Design review of the part built by this model. Coordinates are the model's own, in mm. A direction names the side the tool comes from. Give positions to 0.01 mm unless a question says otherwise; leave off trailing zeros. Write each loop counter-clockwise with the first axis right and the second up, starting at its lowest first coordinate (ties: lowest second). Pieces come first, ordered by that corner, then holes. Notation, with made-up numbers: (88.5, -16) -> (99.5, -16) arc R18 ccw to (99.5, 2) -> close; hole circle Ø1 at (21.25, -24). An arc over 180 degrees is marked (long way). Answer as a JSON object with one key per item and string values.
Autodesk Inventor part; units mm, degrees
ref_plane "Arbeitsebene1" through (-21.4485, 99.4, 5.4) normal (-1, 0, 0) x (0, -0.6026, -0.798)
ref_plane "Arbeitsebene2" through (53.5515, 27.1, 8) normal (0, 0, -1) x (0, 1, 0)
ref_plane "YZ Plane" through (0, 0, 0) normal (1, 0, 0) x (0, 1, 0)
ref_plane "Arbeitsebene1" through (-21.4485, 99.4, 5.4) normal (-1, 0, 0) x (0, -0.6026, -0.798)
sketch "center1" plane through (-21.4485, 99.4, 5.4) normal (-1, 0, 0) x (0, -0.6026, -0.798)
  line L0 (125.8462, -4.4299) -> (-42.8597, 122.9603)
  line L1 (111.6965, 152.237) -> (-23.2865, -26.5243)
  point P0 (64.2081, 76.0713)
ref_plane "Arbeitsebene2" through (53.5515, 27.1, 8) normal (0, 0, -1) x (0, 1, 0)
sketch "center2" plane through (53.5515, 27.1, 8) normal (0, 0, -1) x (0, 1, 0)
  line L0 (0, 239.86) -> (0, -220.81)
  point P0 (-27.1, -53.5515)
sketch "Hallsensor" plane through (0, 0, 0) normal (0, 1, 0) x (-1, 0, 0)
  line L0 (21.4485, 13) -> (41.4485, 13) construction
  line L1 (41.4485, 13) -> (41.4485, 3) construction
  line L2 (41.4485, 3) -> (21.4485, 3) construction
  line L3 (21.4485, 3) -> (21.4485, 13) construction
  line L4 (21.4485, -97.7) -> (21.4485, 113.7) construction
  line L5 (-293.4115, 8) -> (167.2585, 8) construction
  line L6 (40.4485, 4) -> (42.4485, 4)
  line L7 (42.4485, 4) -> (42.4485, 2)
  line L8 (42.4485, 2) -> (40.4485, 2)
  line L9 (40.4485, 2) -> (40.4485, 4)
  line L10 (40.4485, 4) -> (42.4485, 2) construction
  line L11 (42.4485, 4) -> (40.4485, 2) construction
  line L12 (22.4485, 4) -> (20.4485, 4)
  line L13 (20.4485, 4) -> (20.4485, 2)
  line L14 (20.4485, 2) -> (22.4485, 2)
  line L15 (22.4485, 2) -> (22.4485, 4)
  line L16 (22.4485, 4) -> (20.4485, 2) construction
  line L17 (20.4485, 4) -> (22.4485, 2) construction
  line L18 (22.4485, 14) -> (20.4485, 14)
  line L19 (20.4485, 14) -> (20.4485, 12)
  line L20 (20.4485, 12) -> (22.4485, 12)
  line L21 (22.4485, 12) -> (22.4485, 14)
  line L22 (22.4485, 14) -> (20.4485, 12) construction
  line L23 (20.4485, 14) -> (22.4485, 12) construction
  line L24 (42.4485, 14) -> (40.4485, 14)
  line L25 (40.4485, 14) -> (40.4485, 12)
  line L26 (40.4485, 12) -> (42.4485, 12)
  line L27 (42.4485, 12) -> (42.4485, 14)
  line L28 (42.4485, 14) -> (40.4485, 12) construction
  line L29 (40.4485, 14) -> (42.4485, 12) construction
  line L30 (51.4485, -1) -> (1.4485, -1) construction
  line L31 (1.4485, -1) -> (1.4485, 17) construction
  line L32 (1.4485, 17) -> (51.4485, 17) construction
  line L33 (51.4485, 17) -> (51.4485, -1) construction
  circle A0 centre (51.4485, 8) radius 1.5
  circle A1 centre (1.4485, -1) radius 1.5
  circle A2 centre (1.4485, 17) radius 1.5
  point P0 (0, 0)
  point P1 (21.4485, 3)
  point P2 (21.4485, 3)
  dimension "d70" = 20
  dimension "d71" = 10
  dimension "d72" = 2
  dimension "d73" = 4
  dimension "d74" = 4
  dimension "d75" = 20
  dimension "d76" = 10
  dimension "d77" = 3
  dimension "d78" = 5
sketch "Groundplane" plane through (0, 0, 0) normal (0, 1, 0) x (-1, 0, 0)
  line L0 (-293.4115, 8) -> (167.2585, 8) construction
  line L1 (21.4485, -97.7) -> (21.4485, 113.7) construction
  arc A0 (22.4485, -32) -> (20.4485, -32) centre (21.4485, -32) ccw construction
  line L2 (22.4485, -32) -> (20.4485, -32) construction
  line L3 (20.4485, -32) -> (20.4485, -37) construction
  line L4 (20.4485, -37) -> (22.4485, -37) construction
  line L5 (22.4485, -37) -> (22.4485, -32) construction
  arc A1 (20.4485, 48) -> (22.4485, 48) centre (21.4485, 48) ccw construction
  line L6 (20.4485, 48) -> (22.4485, 48) construction
  line L7 (22.4485, 48) -> (22.4485, 53) construction
  line L8 (22.4485, 53) -> (20.4485, 53) construction
  line L9 (20.4485, 53) -> (20.4485, 48) construction
  line L10 (61.4485, -37) -> (-28.5515, -37) construction
  line L11 (-28.5515, -37) -> (-28.5515, 53) construction
  line L12 (-28.5515, 53) -> (61.4485, 53) construction
  line L13 (61.4485, 53) -> (61.4485, -37) construction
  dimension "d87" = 5
  dimension "d88" = 2
  dimension "d89" = 2
  dimension "d90" = 5
  dimension "d91" = 90
  dimension "d92" = 45
  dimension "d97" = 50
  dimension "d98" = 90
sketch "Montagepunkte" plane through (0, 0, 0) normal (0, 1, 0) x (-1, 0, 0)
  circle A0 centre (51.4485, 8) radius 1.5 construction
  circle A1 centre (1.4485, -1) radius 1.5 construction
  circle A2 centre (1.4485, 17) radius 1.5 construction
  line L0 (1.4485, -1) -> (-18.5515, -1) construction
  line L1 (-18.5515, -1) -> (-18.5515, 17) construction
  line L2 (-18.5515, 17) -> (1.4485, 17) construction
  line L3 (1.4485, 17) -> (1.4485, -1) construction
  line L4 (51.4485, 8) -> (31.4485, 8) construction
  circle A3 centre (31.4485, 8) radius 1.6
  circle A4 centre (51.4485, 8) radius 1.6
  circle A5 centre (1.4485, -1) radius 1.6
  circle A6 centre (1.4485, 17) radius 1.6
  circle A7 centre (-18.5515, 17) radius 1.6
  circle A8 centre (-18.5515, -1) radius 1.6
  arc A9 (22.4485, -32) -> (20.4485, -32) centre (21.4485, -32) ccw construction
  arc A10 (20.4485, 48) -> (22.4485, 48) centre (21.4485, 48) ccw construction
  circle A11 centre (21.4485, -32) radius 1
  circle A12 centre (21.4485, 48) radius 1
  dimension "d93" = 20
  dimension "d94" = 20
  dimension "d95" = 3.2
  dimension "d96" = 2
sketch "Skizze5" plane through (0, 0, 0) normal (0, 1, 0) x (-1, 0, 0)
  line L0 (-293.4115, 8) -> (167.2585, 8) construction
  circle A0 centre (21.4485, -32) radius 1
  circle A1 centre (21.4485, 48) radius 1
  line L1 (61.4485, -37) -> (-28.5515, -37)
  line L2 (61.4485, 53) -> (61.4485, -37)
  line L3 (-28.5515, -37) -> (-28.5515, 53)
  line L4 (-28.5515, 53) -> (61.4485, 53)
extrude "Extrusion2" add sketch "Skizze5" along normal blind 5
sketch "Skizze6" plane through (0, 5, 0) normal (0, 1, 0) x (1, 0, 0)
  line L0 (-56.4485, -3) -> (-26.4485, -3)
  line L1 (-26.4485, -3) -> (-26.4485, -13)
  line L2 (-26.4485, -13) -> (-56.4485, -13)
  line L3 (-56.4485, -13) -> (-56.4485, -3)
  line L4 (-6.4485, 6) -> (23.5515, 6)
  line L5 (23.5515, 6) -> (23.5515, -22)
  line L6 (23.5515, -22) -> (-6.4485, -22)
  line L7 (-6.4485, -22) -> (-6.4485, 6)
  circle A0 centre (-51.4485, -8) radius 1.6
  circle A1 centre (-31.4485, -8) radius 1.6
  circle A2 centre (-1.4485, -17) radius 1.6
  circle A3 centre (18.5515, -17) radius 1.6
  circle A4 centre (18.5515, 1) radius 1.6
  circle A5 centre (-1.4485, 1) radius 1.6
  point P0 (0, 0)
  dimension "d99" = 5
  dimension "d100" = 5
  dimension "d101" = 5
  dimension "d102" = 5
  dimension "d103" = 5
  dimension "d104" = 5
  dimension "d105" = 5
  dimension "d106" = 5
extrude "Extrusion3" add sketch "Skizze6" along normal blind 3
chamfer "Fase1" distance 1 distance2 3 2 edges at (-53.0485, 8, 8) (-33.0485, 8, 8) measured on face at (-38.3043, 8, 4.168)
chamfer "Fase2" distance 1 distance2 3 4 edges at (-3.0485, 8, -1) (16.9515, 8, -1) (16.9515, 8, 17) (-3.0485, 8, 17) measured on face at (11.4857, 8, 5.3537)
sketch "Skizze7" plane through (0, 5, 0) normal (0, 1, 0) x (1, 0, 0)
  line L0 (-51.4505, 30) -> (-16.4485, 30)
  line L1 (-13.4485, 27) -> (-13.4485, 7)
  line L2 (-16.4485, 4) -> (-51.4505, 4)
  line L3 (-54.4505, 7) -> (-54.4505, 27)
  line L4 (-51.4505, -20) -> (-16.4485, -20)
  line L5 (-13.4485, -23) -> (-13.4485, -40)
  line L6 (-16.4485, -43) -> (-51.4505, -43)
  line L7 (-54.4505, -40) -> (-54.4505, -23)
  line L8 (-3.4485, -29) -> (18.5497, -29)
  line L9 (21.5497, -32) -> (21.5497, -43)
  line L10 (18.5497, -46) -> (-3.4485, -46)
  line L11 (-6.4485, -43) -> (-6.4485, -32)
  line L12 (28.5497, -53) -> (28.5497, 37)
  line L13 (-61.4505, -53) -> (28.5497, -53)
  line L14 (-61.4505, 37) -> (-61.4505, -53)
  line L15 (-56.4485, -13) -> (-26.4485, -13)
  line L16 (-6.4485, 6) -> (-6.4485, -22)
  line L17 (-26.4485, -3) -> (-56.4485, -3)
  line L18 (28.5497, 37) -> (-61.4505, 37)
  line L19 (-6.4485, -22) -> (23.5515, -22)
  line L20 (-5.4485, 30) -> (20.5497, 30)
  line L21 (21.5497, 29) -> (21.5497, 14)
  line L22 (20.5497, 13) -> (-5.4485, 13)
  line L23 (-6.4485, 14) -> (-6.4485, 29)
  line L24 (23.5515, 6) -> (-6.4485, 6)
  arc A0 (-51.4505, 30) -> (-54.4505, 27) centre (-51.4505, 27) ccw
  arc A1 (-54.4505, 7) -> (-51.4505, 4) centre (-51.4505, 7) ccw
  arc A2 (-13.4485, 27) -> (-16.4485, 30) centre (-16.4485, 27) ccw
  arc A3 (-16.4485, 4) -> (-13.4485, 7) centre (-16.4485, 7) ccw
  arc A4 (-51.4505, -20) -> (-54.4505, -23) centre (-51.4505, -23) ccw
  arc A5 (-13.4485, -23) -> (-16.4485, -20) centre (-16.4485, -23) ccw
  arc A6 (-16.4485, -43) -> (-13.4485, -40) centre (-16.4485, -40) ccw
  arc A7 (-54.4505, -40) -> (-51.4505, -43) centre (-51.4505, -40) ccw
  arc A8 (-3.4485, -29) -> (-6.4485, -32) centre (-3.4485, -32) ccw
  arc A9 (-6.4485, -43) -> (-3.4485, -46) centre (-3.4485, -43) ccw
  arc A10 (18.5497, -46) -> (21.5497, -43) centre (18.5497, -43) ccw
  arc A11 (21.5497, -32) -> (18.5497, -29) centre (18.5497, -32) ccw
  arc A12 (-5.4485, 30) -> (-6.4485, 29) centre (-5.4485, 29) ccw
  arc A13 (-6.4485, 14) -> (-5.4485, 13) centre (-5.4485, 14) ccw
  arc A14 (21.5497, 29) -> (20.5497, 30) centre (20.5497, 29) ccw
  arc A15 (20.5497, 13) -> (21.5497, 14) centre (20.5497, 14) ccw
  point P0 (0, 0)
  point P1 (-13.4485, -43)
  point P2 (-41.4485, -3)
  point P3 (-6.4485, -37.5)
  point P4 (-6.4485, 21.5)
  dimension "d42" = 7
  dimension "d43" = 7
  dimension "d44" = 7
  dimension "d45" = 10
  dimension "d46" = 7
  dimension "d47" = 7
  dimension "d48" = 7
  dimension "d49" = 7
  dimension "d50" = 7
  dimension "d51" = 7
  dimension "d52" = 7
  dimension "d53" = 7
  dimension "d54" = 7
  dimension "d55" = 7
  dimension "d56" = 7
  dimension "d57" = 7
  dimension "d58" = 3
  dimension "d59" = 3
  dimension "d60" = 1
extrude "Extrusion4" cut sketch "Skizze7" against normal through all contours L0 A2 L1 A3 L2 A1 L3 A0 | L4 A5 L5 A6 L6 A7 L7 A4 | L8 A11 L9 A10 L10 A9 L11 A8 | L20 A14 L21 A15 L22 A13 L23 A12
sketch "Skizze11" plane through (0, 5, 0) normal (0, 1, 0) x (1, 0, 0)
  line L0 (-54.4505, 7) -> (-54.4505, 27)
  line L1 (-13.4485, 27) -> (-13.4485, 7)
  line L2 (20.5497, 13) -> (-5.4485, 13) construction
  line L3 (-54.4505, 18) -> (-43.4485, 22)
  line L4 (-43.4485, 22) -> (-43.4485, 19)
  line L5 (-43.4485, 19) -> (-13.4485, 19)
  line L6 (-54.4505, 16) -> (-43.4485, 12)
  line L7 (-43.4485, 12) -> (-43.4485, 15)
  line L8 (-43.4485, 15) -> (-13.4485, 15)
  line L9 (14.239, 13) -> (11.6491, 13)
  line L10 (11.6491, 13) -> (7.5162, 19.778)
  line L11 (7.5162, 19.778) -> (3.3006, 13)
  line L12 (3.3006, 13) -> (0.8622, 13)
  line L13 (0.8622, 13) -> (6.2763, 21.5138)
  line L14 (6.2763, 21.5138) -> (1.0275, 30)
  line L15 (1.0275, 30) -> (3.6175, 30)
  line L16 (3.6175, 30) -> (7.6677, 23.346)
  line L17 (7.6677, 23.346) -> (11.8006, 30)
  line L18 (11.8006, 30) -> (14.239, 30)
  line L19 (14.239, 30) -> (8.9214, 21.624)
  line L20 (8.9214, 21.624) -> (14.239, 13)
  point P0 (0, 0)
  point P1 (-54.4505, 17)
  point P2 (-54.4505, 17)
  point P3 (-54.4505, 17)
  point P4 (-54.4505, 17)
  point P5 (-54.4505, 17)
  dimension "d108" = 4
  dimension "d109" = 2
  dimension "d110" = 30
  dimension "d111" = 3
  dimension "d112" = 3
  dimension "d113" = 1
  dimension "d114" = 1
extrude "Extrusion5" add sketch "Skizze11" against normal up to surface (5 mm away)
properties part number "HallSensor_Halterung"
(1) For line 1 along Z through (x, y) = (-42, 2.75); line 2 along Z through (x, y) = (-4, 2); line 3 along Z through (x, y) = (-1.5, 3), list the stretches that pass through material, from the lowest coordinate up.
Here are the results:
{"line 1": "z = -37 to -30, -19 to -15, -4 to 20, 43 to 53", "line 2": "z = -37 to -30, -13 to 29.05, 45.95 to 53", "line 3": "z = -37 to -30, -13 to 29, 46 to 53"}
(2) We need section B-B, the plane z = 41.5. State the section outline as (x, y) points.
Here are the results:
{"outline": "(-61.45, 0) -> (-54.05, 0) -> (-54.05, 5) -> (-61.45, 5) -> close; (-13.85, 0) -> (-6.45, 0) -> (-6.45, 5) -> (-13.85, 5) -> close; (21.55, 0) -> (28.55, 0) -> (28.55, 5) -> (21.55, 5) -> close"}
(3) For faces 1 (the flat face through (9, 6, 22)), 2 (the flat face through (-13.448, 3, -23)), 3 (the flat face through (8, 6, -6)), 4 (the flat face through (-41, 6, 13)), list the 3-axis set-ups (+Z, -Z, +X, -X, +Y, -Y) from which the entire face can be reached by the end or side of a thin tool; tool diameter is ignored.
Here are the results:
{"face 1": "+Z, +X, -X, +Y", "face 2": "+Y, -Y", "face 3": "-Z, +X, -X, +Y", "face 4": "+Z, -X, +Y"}
(4) The part is to be moulded in two halves that separate along X. For faces 5 (the flat face through (8, 8, 8)), 6 (the flat face through (-61.448, 2, 9)), 7 (the flat face through (5.44, 2.54, -16.44)), say which applies: +X half, -X half, draft (parallel to the pull), parting line (faces both ways), or undercut.
Here are the results:
{"face 5": "draft", "face 6": "-X half", "face 7": "undercut"}
(5) We need section C-C, the plane y = 3.25. Give the number of separate pieces and of enclosed holes in the cut face, then the cut area to 3 significant figures.
Here are the results:
{"separate pieces": "1", "enclosed holes": "10", "area": "5,420 mm²"}
(6) Clearance check with flat-ended pins moving along their axes: pin 1 (1.5 mm diameter, centred on y = 6.5, z = 5.5, fed in from -X); pin 2 (2.5 mm diameter, centred on x = -38, y = 6.5, fed in from +Z); pin 3 (10 mm diameter, centred on x = -37, z = 34, fed in from +Y); pin 4 (2.5 mm diameter, centred on x = -21.45, z = 48, fed in from +Y). State where each tip first meets the part, or that it passes through.
Here are the results:
{"pin 1": "stops at x = -56.45", "pin 2": "stops at z = 13", "pin 3": "passes through", "pin 4": "stops at y = 5"}
